Can you work these out from the model? Positions are in its coordinate system, mm. Coordinates: 2 decimals unless noted, no trailing zeros. Order: outer loops, then holes, each group sorted by start corner. A loop starts at its lowest first (then second) coordinate and runs counter-clockwise, first axis right, second up. Notation, with made-up numbers: (74, 30.25) -> (91, 30.25) arc R16 cw to (91, 61.25) -> close; hole circle Ø8 at (40, -25). An arc over 180 degrees is marked (long way). Answer in a Markdown table with one row per item.
```python
from build123d import *

# Parameters (mm, degrees)
F0_W          = 25
F0_H          = 25
F1_DEPTH      = 1700
F3_DEPTH      = 12.501
F3_DEPTH_BACK = 12.501
F5_DEPTH      = 12.501
F5_DEPTH_BACK = 12.501


with BuildPart() as f1:
    # F0 (on Right) → F1 (new body)
    with BuildSketch(Plane.YZ):
        Rectangle(F0_W, F0_H)
    extrude(amount=F1_DEPTH)

    # F2 (on Front) → F3 (cut, two sides)
    with BuildSketch(Plane.XZ) as f3_sk:
        Polygon((25, -12.5), (0, 12.5), (0, -12.5), align=None)
    extrude(amount=-F3_DEPTH, mode=Mode.SUBTRACT)
    extrude(f3_sk.sketch, amount=F3_DEPTH_BACK, mode=Mode.SUBTRACT)

    # F4 (on Front) → F5 (cut, two sides)
    with BuildSketch(Plane.XZ) as f5_sk:
        Polygon((1700, -12.5), (1700, 12.5), (1675, -12.5), align=None)
    extrude(amount=-F5_DEPTH, mode=Mode.SUBTRACT)
    extrude(f5_sk.sketch, amount=F5_DEPTH_BACK, mode=Mode.SUBTRACT)


solid = f1.part
```
(1) Will these pins go through, and if not, where does the flat tip stop? pin 1 Ø8 at (y, z) = (0.5, 3.5) entering from +X; pin 2 Ø10 at (y, z) = (-1.5, -3.5) entering from +X; pin 3 Ø8 at (y, z) = (9.5, 3) entering from +X.
Response values:
| item | result |
|---|---|
| pin 1 | x = 1695 |
| pin 2 | x = 1689 |
| pin 3 | x = 1694.5 |
(2) Suppose I cut it at A-A (z = -7.5). Please give me the cut outline in (x, y).
Response values:
| item | result |
|---|---|
| outline | (20, -12.5) -> (1680, -12.5) -> (1680, 12.5) -> (20, 12.5) -> close |
(3) I need wall thicknesses on line 1 (X direction, y = 2, z = 7.5); line 2 (X direction, y = -4.25, z = -5.25). Which ranges of each line are inside material? Lowest first, please. Write a range as [from, to].
Response values:
| item | result |
|---|---|
| line 1 | [5, 1695] |
| line 2 | [17.75, 1682.25] |
